Read the model definition and answer for the solid it produces. Units are mm, in the model's axes. Face numbers are marked on the shaded views. A direction names the side the tool comes from. Give positions to 0.01 mm unless a question says otherwise; leave off trailing zeros. Loops run counter-clockwise (first coordinate to the right, second up) from the corner with the lowest first, then second, coordinate; pieces in that order, holes last.
(1) Find section A-A, the plane z = 51. Write down the section's boundary in (x, y), then the cut area to 3 significant figures.
(2) Which of the six approach directions +Z, -Z, +X, -X, +Y, -Y give full straight-line access (tool end or side, diameter ignored) to the marked faces 1 and 2?
(3) Find section D-D, the plane z = 13.5. Write down the section's boundary in (x, y).
(4) Each of these flat-tipped pins is pushed along its axis until it touches: P1, Ø5, axis at y = 11, z = 20.5, coming from the +X side; P2, Ø1.5, axis at y = 13.5, z = 14.5, coming from the -X side. Where does it stop, or does it pass through?
(5) Find section B-B, the plane x = 15. Write down the section's boundary in (y, z).
(6) Straight lines are drawn through the part: probe 1 along Y at (x, z) = (2, 6); probe 2 along X at (y, z) = (8.5, 43). For each, find the intervals that lie inside material, in ascending order.
Autodesk Inventor part; units mm, degrees
ref_plane "YZ Plane" through (0, 0, 0) normal (1, 0, 0) x (0, 1, 0)
ref_plane "XZ Plane" through (0, 0, 0) normal (0, 1, 0) x (-1, 0, 0)
ref_plane "XY Plane" through (0, 0, 0) normal (0, 0, 1) x (1, 0, 0)
sketch "Sketch1" plane through (0, 0, 0) normal (0, 0, 1) x (1, 0, 0)
  line L0 (0, 0) -> (0, 20)
  line L1 (0, 20) -> (3, 20)
  line L2 (3, 20) -> (3, 3)
  line L3 (3, 3) -> (20, 3)
  line L4 (20, 3) -> (20, 0)
  line L5 (20, 0) -> (0, 0)
  dimension "d0" = 20
  dimension "d1" = 3
  dimension "d2" = 17
  dimension "d3" = 17
extrude "Extrusion1" add sketch "Sketch1" along normal blind 59.6
sketch "Sketch2" plane through (3, 3, 0) normal (0, 1, 0) x (1, 0, 0)
  line L0 (0, 0) -> (17, 0)
  line L1 (17, -59.6) -> (0, -59.6)
  line L2 (17, 0) -> (17, -59.6)
  line L3 (12, -59.6) -> (12, 0) construction
  line L4 (12, -12.55) -> (12, -12.55)
  line L5 (9.25, -9.8) -> (9.25, -4.8)
  line L6 (12, -2.05) -> (12, -2.05)
  line L7 (14.75, -4.8) -> (14.75, -9.8)
  line L8 (14.75, -12.55) -> (9.25, -2.05) construction
  line L9 (9.25, -12.55) -> (14.75, -2.05) construction
  arc A0 (9.25, -9.8) -> (12, -12.55) centre (12, -9.8) ccw
  arc A1 (12, -12.55) -> (14.75, -9.8) centre (12, -9.8) ccw
  arc A2 (14.75, -4.8) -> (12, -2.05) centre (12, -4.8) ccw
  arc A3 (12, -2.05) -> (9.25, -4.8) centre (12, -4.8) ccw
  point P0 (-3, 0)
  point P1 (12, -7.3)
  dimension "bottom_row_offset" = 5
  dimension "d7" = 5.5
  dimension "hole_length" = 10.5
  dimension "bottom_hole_edge_offset" = 2.05
  dimension "d10" = 2.75
extrude "Extrusion2" cut sketch "Sketch2" against normal through all
sketch "Sketch3" plane through (3, 3, 0) normal (1, 0, 0) x (0, 0, -1)
  line L0 (0, 17) -> (0, 0)
  line L1 (0, 17) -> (-59.6, 17)
  line L2 (-59.6, 0) -> (-59.6, 17)
  line L3 (-59.6, 7) -> (0, 7) construction
  line L4 (-9.8, 9.75) -> (-4.8, 9.75)
  line L5 (-2.05, 7) -> (-2.05, 7)
  line L6 (-4.8, 4.25) -> (-9.8, 4.25)
  line L7 (-12.55, 7) -> (-12.55, 7)
  line L8 (-12.55, 9.75) -> (-2.05, 4.25) construction
  line L9 (-2.05, 9.75) -> (-12.55, 4.25) construction
  arc A0 (-9.8, 9.75) -> (-12.55, 7) centre (-9.8, 7) ccw
  arc A1 (-12.55, 7) -> (-9.8, 4.25) centre (-9.8, 7) ccw
  arc A2 (-4.8, 4.25) -> (-2.05, 7) centre (-4.8, 7) ccw
  arc A3 (-2.05, 7) -> (-4.8, 9.75) centre (-4.8, 7) ccw
  point P0 (0, -3)
  point P1 (-7.3, 7)
  dimension "top_row_offset" = 10
  dimension "d14" = 10.5
  dimension "d15" = 5.5
  dimension "d16" = 2.75
  dimension "d17" = 2.05
extrude "Extrusion3" cut sketch "Sketch3" against normal through all
pattern_linear "Rectangular Pattern1" count 3 spacing 22.5 along (0, 0, 1) of "Extrusion2", "Extrusion3"
equation "\"d14\" = hole_length"
equation "\"d17\" = bottom_hole_edge_offset"
equation "\"hole_number\" = 3"
properties part number "Universal L Bracket" material "Aluminum 6061"
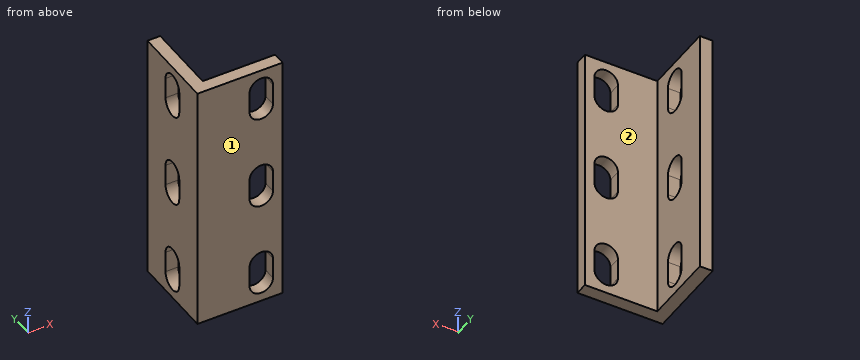
Entries:
1. outline: (0, 0) - (12.25, 0) - (12.25, 3) - (3, 3) - (3, 7.25) - (0, 7.25) - close; (0, 12.75) - (3, 12.75) - (3, 20) - (0, 20) - close; (17.75, 0) - (20, 0) - (20, 3) - (17.75, 3) - close
1. area: 78.0 mm2
2. face 1: +Z, -Z, +X, -X, -Y
2. face 2: +Z, -Z, +X, +Y
3. outline: (0, 0) - (20, 0) - (20, 3) - (3, 3) - (3, 20) - (0, 20) - close
4. P1: stops at x = 3
4. P2: stops at x = 0
5. outline: (0, 0) - (3, 0) - (3, 2.05) - (0, 2.05) - close; (0, 12.55) - (3, 12.55) - (3, 24.55) - (0, 24.55) - close; (0, 35.05) - (3, 35.05) - (3, 47.05) - (0, 47.05) - close; (0, 57.55) - (3, 57.55) - (3, 59.6) - (0, 59.6) - close
6. probe 1: y = 0 to 7.25, 12.75 to 20
6. probe 2: x = 0 to 3
